Part model, mm, in its own coordinate system. A direction names the side the tool comes from. Round coordinates to 2 decimals unless told otherwise and drop trailing zeros. Write each loop counter-clockwise with the first axis right and the second up, starting at its lowest first coordinate (ties: lowest second). Pieces come first, ordered by that corner, then holes. Notation, with made-up numbers: M -8,25.25 L 13,25.25 A17 ccw 13,37.25 Z; hole C 5.5,66.5 d6. An arc over 180 degrees is marked long. Use a Markdown table: item, result. Add a question column.
1) Drop flat-ended pins along their axis: P1, Ø1.5, axis at y = 2.5, z = 2, coming from the -X side; P2, Ø19.5, axis at x = -0.5, y = 1.5, coming from the +Z side; P3, Ø3, axis at x = -9.5, z = 3, coming from the -Y side. Give the stop position or say it passes through.
2) Which spindle directions (+Z, -Z, +X, -X, +Y, -Y) get a long thin tool onto all of the face, cutting with end or side? Do faces 1 (the face through (9.247, -39.525, 1.521)), 2 (the face through (-4, -33, 3)), 3 (the face through (9, -9, 4)). Say none if no direction does.
3) Wall check: probe 1 along Y at (x, z) = (0, 1.15); probe 2 along Y at (x, z) = (0, 3.6); probe 3 along X at (y, z) = (-41, 5.75). Give the ranges that are in metal, low to high.
4) Slice it at A-A on x = 0. Write the cut outline in (y, z), plus the area to 3 significant figures.
5) Two-plate mould, pull along X, no slides. Class faces 4 (the face through (-14, -5, 2)), 5 (the face through (-9, -9, 4)), 6 (the face through (0, 13.924, 1)): released by +X, released by -X, zero draft, split by the parting line, or undercut.
6) Slice it at C-C on y = -2. Write the cut outline in (x, z), plus the area to 3 significant figures.
7) Slice it at B-B on z = 1.25. Write the cut outline in (x, y).
Autodesk Inventor part; units mm, degrees
ref_plane "YZ Plane" through (0, 0, 0) normal (1, 0, 0) x (0, 1, 0)
ref_plane "XZ Plane" through (0, 0, 0) normal (0, 1, 0) x (-1, 0, 0)
ref_plane "XY Plane" through (0, 0, 0) normal (0, 0, 1) x (1, 0, 0)
sketch "Sketch1" plane through (0, 0, 0) normal (0, 0, 1) x (1, 0, 0)
  line L0 (-14, 13.9238) -> (14, 13.9238)
  line L1 (14, 13.9238) -> (14, -13.9238)
  line L2 (14, -29.5762) -> (-14, -29.5762)
  line L3 (-14, -29.5762) -> (-14, -13.9238)
  arc A0 (-14, -13.9238) -> (14, -13.9238) centre (0, -29.5762) ccw
  line L4 (-14, -13.9238) -> (-14, 13.9238)
  line L5 (14, -13.9238) -> (14, -29.5762)
  point P0 (0, 0)
  point P1 (0, 13.9238)
  point P2 (14, 0)
  dimension "d0" = 42
  dimension "d1" = 43.5
  dimension "d4" = 28
extrude "Extrusion1" add sketch "Sketch1" along normal blind 3
sketch "Sketch2" plane through (0, 0, 3) normal (0, 0, 1) x (1, 0, 0)
  line L0 (14, -13.9238) -> (14, 13.9238)
  line L1 (14, 13.9238) -> (-14, 13.9238) construction
  line L2 (-14, 13.9238) -> (-14, -13.9238) construction
  arc A0 (-14, -13.9238) -> (14, -13.9238) centre (0, -29.5762) ccw
  circle A1 centre (0, -29.5762) radius 16.75
  circle A2 centre (0, -29.5762) radius 21
  line L3 (-14, -6.0762) -> (14, -6.0762)
  line L4 (14, -13.9238) -> (14, 13.9238) construction
  line L5 (-14, 13.9238) -> (-14, -13.9238)
  line L6 (-14, -6.0762) -> (-14, -13.9238)
  line L7 (-9, -6.0762) -> (-9, -10.6026)
  line L8 (14, -6.0762) -> (14, -13.9238)
  line L9 (9, -10.6026) -> (9, -6.0762)
  arc A3 (-14, -13.9238) -> (14, -13.9238) centre (0, -29.5762) ccw
  line L10 (14, -6.0762) -> (14, -13.9238)
  point P0 (0, 0)
  dimension "d5" = 33.5
  dimension "d6" = 20
  dimension "d7" = 5
  dimension "d8" = 5
extrude "Extrusion2" add sketch "Sketch2" along normal blind 3 contours A2 L9 L3 L0 | A0 A2 | L5 L3 L7 A2
sketch "Sketch3" plane through (0, 0, 3) normal (0, 0, 1) x (1, 0, 0)
  circle A0 centre (0, -29.5762) radius 16.75
  circle A1 centre (0, -29.5762) radius 5
  line L0 (9, -6.0762) -> (14, -6.0762)
  line L1 (14, -6.0762) -> (14, 13.9238)
  line L2 (14, 13.9238) -> (-14, 13.9238)
  line L3 (-14, 13.9238) -> (-14, -6.0762)
  line L4 (-14, -6.0762) -> (-9, -6.0762)
  line L5 (-9, -6.0762) -> (-9, -10.6026)
  arc A2 (9, -10.6026) -> (-9, -10.6026) centre (0, -29.5762) ccw
  line L6 (9, -10.6026) -> (9, -6.0762)
  circle A3 centre (-6, 3.9238) radius 2.1
  circle A4 centre (6, 3.9238) radius 2.1
  line L7 (-6, 3.9238) -> (6, 3.9238) construction
  point P0 (0, 0)
  point P1 (0, 3.9238)
  dimension "d11" = 10
  dimension "d12" = 4.2
  dimension "d13" = 12
  dimension "d14" = 10
extrude "Extrusion3" cut sketch "Sketch3" against normal up to next contours A1 | A3 | A4
chamfer "Chamfer1" distance 3 angle 45 2 edges at (11.5, -6.0762, 6) (-11.5, -6.0762, 6)
fillet "Fillet1" radius 1 7 edges at (-16.75, -29.5762, 6) (0, -8.5762, 6) (0, -50.5762, 6) (-14, -11.4998, 6) (-9, -9.8392, 6) (9, -9.8392, 6) (14, -11.4998, 6)
sketch "Sketch4" plane through (0, -29.5762, 3) normal (0, 0, 1) x (1, 0, 0)
  circle A0 centre (0, 0) radius 5
  circle A1 centre (8.4853, 8.4853) radius 1.65
  line L0 (0, 0) -> (8.4853, 8.4853) construction
  line L1 (0, 0) -> (0, 12.1192) construction
  line L2 (0, 0) -> (-12.1192, 0) construction
  circle A2 centre (-8.4853, 8.4853) radius 1.65
  line L3 (0, 0) -> (0, -12.1192) construction
  circle A3 centre (-8.4853, -8.4853) radius 1.65
  line L4 (0, 0) -> (12.1192, 0) construction
  circle A4 centre (8.4853, -8.4853) radius 1.65
  point P0 (0, 29.5762)
  dimension "d21" = 45
  dimension "d22" = 3.3
  dimension "d23" = 12
  dimension "d26" = 360
extrude "Extrusion4" cut sketch "Sketch4" against normal up to next contours A1 | A2 | A3 | A4
fillet "Fillet2" radius 4 2 edges at (-14, 13.9238, 1.5) (14, 13.9238, 1.5)
equation "\"d8\" = d7"
properties part number "holder-LMF8LUU-z-axis"
Entries:
| question | item | result |
|---|---|---|
| 1 | P1 | stops at x = -14 |
| 1 | P2 | stops at z = 3 |
| 1 | P3 | stops at y = -48.99 |
| 2 | face 1 | +Z, -Z |
| 2 | face 2 | +Z |
| 2 | face 3 | +Z, +Y |
| 3 | probe 1 | y = -50.58 to -34.58, -24.58 to 13.92 |
| 3 | probe 2 | y = -50.58 to -46.33, -12.83 to -8.58 |
| 3 | probe 3 | x = -17.22 to -12.71, 12.71 to 17.22 |
| 4 | outline | M -50.58,0 L -34.58,0 L -34.58,3 L -46.33,3 L -46.33,5 A1 ccw -47.33,6 L -49.58,6 A1 ccw -50.58,5 Z; M -24.58,0 L 13.92,0 L 13.92,3 L -8.58,3 L -8.58,5 A1 ccw -9.58,6 L -11.83,6 A1 ccw -12.83,5 L -12.83,3 L -24.58,3 Z |
| 4 | area | 188 mm^2 |
| 5 | face 4 | released by -X |
| 5 | face 5 | undercut |
| 5 | face 6 | zero draft |
| 6 | outline | M -14,0 L 14,0 L 14,3 L -14,3 Z |
| 6 | area | 84.0 mm^2 |
| 7 | outline | M -14,-13.92 A21 ccw long 14,-13.92 L 14,9.92 A4 ccw 10,13.92 L -10,13.92 A4 ccw -14,9.92 Z; hole C -8.49,-38.06 d3.3; hole C -8.49,-21.09 d3.3; hole C -6,3.92 d4.2; hole C 0,-29.58 d10; hole C 6,3.92 d4.2; hole C 8.49,-38.06 d3.3; hole C 8.49,-21.09 d3.3 |
